Can you work these out from the model? Positions are in its coordinate system, mm. A direction names the side the tool comes from. Round coordinates to 2 decimals unless told otherwise and drop trailing zeros. Write each loop counter-clockwise with the first axis right and the second up, starting at its lowest first coordinate (ties: lowest second). Pieces come first, ordered by that corner, then holes. Notation, with made-up numbers: M 20,22 L 76,22 A3 cw 76,26 Z; hole C 54,53.25 d9. An arc over 180 degrees is marked long. Answer in a Markdown table with one row per item. Add a question column.
(1) Suppose I cut it at A-A, the plane z = 0. Write out the boundary of the cut face in (x, y), then the cut area to 3 significant figures.
(2) Suppose I cut it at D-D, the plane x = -1. Write out the boundary of the cut face in (y, z).
(3) If I drill on probe 1 along Y at (x, z) = (-37.5, 4); probe 2 along X at (y, z) = (-29, 13.5); probe 3 along X at (y, z) = (65, -5), over which ranges is the centre line in solid material (lowest first)?
(4) Suppose I cut it at C-C, the plane y = -27. Write out the boundary of the cut face in (x, z).
(5) I'm going to push flat-ended pins straight in: pin 1 (1.8 mm diameter, centred on x = -2, y = 74, fed in from +Z); pin 2 (3 mm diameter, centred on x = -27.5, z = 5.5, fed in from -Y); pin 3 (6.5 mm diameter, centred on x = -44, y = -30.5, fed in from +Z); pin 4 (12 mm diameter, centred on x = -20.5, z = 24.5, fed in from -Y). Where does each tip first touch, or does it pass through?
(6) For faces 1 (the face through (-40, -13, 15.25)), 2 (the face through (-35, 10.571, 0)), 3 (the face through (-12, -13.5, 0)), which set-ups out of +Z, -Z, +X, -X, +Y, -Y let a thin tool reach every point of the face, with its end or its side?
(7) If we mould it in two halves opening along Z, with no side actions, what happens to faces 4 (the face through (-46, -26, -13.75)), 5 (the face through (-33, -25, 0)), 6 (the face through (0, 74, 10))? For each: released by +Z, released by -Z, zero draft, split by the parting line, or undercut.
(8) Suppose I cut it at B-B, the plane x = -49. Write out the boundary of the cut face in (y, z), then the cut area to 3 significant figures.
from build123d import *

# Parameters (mm, degrees)
SKETCH1_W            = 15
SKETCH1_H            = 18.5
BOSS_EXTRUDE1_DEPTH  = 10
SKETCH3_W            = 60
SKETCH3_H            = 24.642135624
BOSS_EXTRUDE2_DEPTH  = 20
BOSS_EXTRUDE3_DEPTH  = 20
SKETCH5_R            = 5.1
CUT_EXTRUDE1_DEPTH   = 120.21693154
SKETCH6_W            = 15
SKETCH6_H            = 18.5
BOSS_EXTRUDE4_DEPTH  = 50
BOSS_EXTRUDE5_DEPTH  = 25
SKETCH8_W            = 3
SKETCH8_H            = 30.5
BOSS_EXTRUDE6_DEPTH  = 25
SKETCH9_W            = 25
SKETCH9_H            = 1.5
BOSS_EXTRUDE7_DEPTH  = 22
BOSS_EXTRUDE11_START = 2
BOSS_EXTRUDE11_DEPTH = 2


with BuildPart() as part:
    # Sketch1 → Boss-Extrude1 (new, symmetric)
    with BuildSketch(Plane.YZ):
        with BuildLine():
            Line((13.5, 5.25), (13.5, -5.25))
            ThreePointArc((13.5, -5.25), (10.571067812, -12.321067812), (3.5, -15.25))
            Line((3.5, -15.25), (-3.5, -15.25))
            ThreePointArc((-3.5, -15.25), (-10.571067812, -12.321067812), (-13.5, -5.25))
            Line((-13.5, -5.25), (-13.5, 5.25))
            ThreePointArc((-13.5, 5.25), (-10.571067812, 12.321067812), (-3.5, 15.25))
            Line((-3.5, 15.25), (3.5, 15.25))
            ThreePointArc((3.5, 15.25), (10.571067812, 12.321067812), (13.5, 5.25))
        make_face()
        Rectangle(SKETCH1_W, SKETCH1_H, mode=Mode.SUBTRACT)
    extrude(amount=BOSS_EXTRUDE1_DEPTH, both=True)

    # Sketch3 → Boss-Extrude2 (add)
    with BuildSketch(Plane.YZ.offset(10)):
        with Locations((40.571067812, 0)):
            Rectangle(SKETCH3_W, SKETCH3_H)
    extrude(amount=-BOSS_EXTRUDE2_DEPTH)

    # Sketch4 → Boss-Extrude3 (add)
    with BuildSketch(Plane.YZ.offset(10)):
        Polygon((70.571067812, 10), (76.571067812, 10), (76.571067812, 45), (108.571067812, 45), (108.571067812, -45), (76.571067812, -45), (76.571067812, -10), (70.571067812, -10), align=None)
    extrude(amount=-BOSS_EXTRUDE3_DEPTH)

    # Sketch5 → Cut-Extrude1 (cut, through all)
    with BuildSketch(Plane.YZ.offset(10)):
        with Locations(Location((95.921067812, 0, 0), (0, 0, 270))):
            Circle(SKETCH5_R)
    extrude(amount=-CUT_EXTRUDE1_DEPTH, mode=Mode.SUBTRACT)

    # Sketch6 → Boss-Extrude4 (add)
    with BuildSketch(Plane(origin=(-10, 0, 0), x_dir=(0, -1, 0), z_dir=(-1, 0, 0))):
        with BuildLine():
            Line((-10.571067812, 12.321067812), (-10.571067812, -12.321067812))
            ThreePointArc((-10.571067812, -12.321067812), (-7.326834324, -14.488795325), (-3.5, -15.25))
            Line((-3.5, -15.25), (3.5, -15.25))
            ThreePointArc((3.5, -15.25), (10.571067812, -12.321067812), (13.5, -5.25))
            Line((13.5, -5.25), (13.5, 5.25))
            ThreePointArc((13.5, 5.25), (10.571067812, 12.321067812), (3.5, 15.25))
            Line((3.5, 15.25), (-3.5, 15.25))
            ThreePointArc((-3.5, 15.25), (-7.326834324, 14.488795325), (-10.571067812, 12.321067812))
        make_face()
        Rectangle(SKETCH6_W, SKETCH6_H, mode=Mode.SUBTRACT)
    extrude(amount=BOSS_EXTRUDE4_DEPTH)

    # Sketch7 → Boss-Extrude5 (add)
    with BuildSketch(Plane(origin=(-60, 0, 0), x_dir=(0, -1, 0), z_dir=(-1, 0, 0))):
        Polygon((3.5, 15.25), (13.5, 15.25), (13.5, -15.25), (3.5, -15.25), (3.5, -9.25), (7.5, -9.25), (7.5, 9.25), (3.5, 9.25), align=None)
    extrude(amount=-BOSS_EXTRUDE5_DEPTH)

    # Sketch8 → Boss-Extrude6 (add)
    with BuildSketch(Plane.XZ.offset(13.5)):
        with Locations((-58.5, 0)):
            Rectangle(SKETCH8_W, SKETCH8_H)
    extrude(amount=BOSS_EXTRUDE6_DEPTH)

    # Sketch9 → Boss-Extrude7 (add)
    with BuildSketch(Plane.YZ.offset(-57)):
        with Locations((-26, 14.5)):
            Rectangle(SKETCH9_W, SKETCH9_H)
        with Locations((-26, -14.5)):
            Rectangle(SKETCH9_W, SKETCH9_H)
    extrude(amount=BOSS_EXTRUDE7_DEPTH)

    # Sketch10 → Boss-Extrude11 (add)
    with BuildSketch(Plane.YZ.offset(-35).offset(BOSS_EXTRUDE11_START)):
        with BuildLine():
            Line((-3.5, 15.25), (-38.5, 15.25))
            Line((-38.5, 15.25), (-38.5, 13.75))
            Line((-38.5, 13.75), (-13.5, 13.75))
            Line((-13.5, 13.75), (-13.5, 5.25))
            ThreePointArc((-13.5, 5.25), (-10.571067812, 12.321067812), (-3.5, 15.25))
        make_face()
        Polygon((-13.5, 13.75), (-38.5, 13.75), (-38.5, -13.75), (-13.5, -13.75), (-13.5, -5.25), (-13.5, 5.25), align=None)
        with BuildLine():
            Line((-13.5, -13.75), (-38.5, -13.75))
            Line((-38.5, -13.75), (-38.5, -15.25))
            Line((-38.5, -15.25), (-3.5, -15.25))
            ThreePointArc((-3.5, -15.25), (-10.571067812, -12.321067812), (-13.5, -5.25))
            Line((-13.5, -5.25), (-13.5, -13.75))
        make_face()
    extrude(amount=-BOSS_EXTRUDE11_DEPTH)


solid = part.part
Calculated:
| question | item | result |
|---|---|---|
| 1 | outline | M -60,-38.5 L -57,-38.5 L -57,-13.5 L -35,-13.5 L -35,-38.5 L -33,-38.5 L -33,-13.5 L 10,-13.5 L 10,-7.5 L -60,-7.5 Z; M -60,7.5 L 10,7.5 L 10,90.82 L -10,90.82 L -10,10.57 L -60,10.57 Z; M -10,101.02 L 10,101.02 L 10,108.57 L -10,108.57 Z |
| 1 | area | 2,520 mm² |
| 2 | outline | M -13.5,-5.25 A10 ccw -3.5,-15.25 L 3.5,-15.25 A10 ccw 10.57,-12.32 L 70.57,-12.32 L 70.57,-10 L 76.57,-10 L 76.57,-45 L 108.57,-45 L 108.57,45 L 76.57,45 L 76.57,10 L 70.57,10 L 70.57,12.32 L 10.57,12.32 A10 ccw 3.5,15.25 L -3.5,15.25 A10 ccw -13.5,5.25 Z; hole M -7.5,-9.25 L 7.5,-9.25 L 7.5,9.25 L -7.5,9.25 Z; hole C 95.92,0 d10.2 |
| 3 | probe 1 | -13.5 to -7.5, 7.5 to 10.57 |
| 3 | probe 2 | -60 to -57, -35 to -33 |
| 3 | probe 3 | -10 to 10 |
| 4 | outline | M -60,-15.25 L -33,-15.25 L -33,15.25 L -60,15.25 Z; hole M -57,-13.75 L -35,-13.75 L -35,13.75 L -57,13.75 Z |
| 5 | pin 1 | z = 10 |
| 5 | pin 2 | y = -13.5 |
| 5 | pin 3 | z = 15.25 |
| 5 | pin 4 | through |
| 6 | face 1 | +Z, +X, -X, -Y |
| 6 | face 2 | +Z, -Z, -X, +Y |
| 6 | face 3 | +Z, -Z, +X, -Y |
| 7 | face 4 | undercut |
| 7 | face 5 | zero draft |
| 7 | face 6 | released by +Z |
| 8 | outline | M -38.5,-15.25 L 3.5,-15.25 A10 ccw 10.57,-12.32 L 10.57,12.32 A10 ccw 3.5,15.25 L -38.5,15.25 L -38.5,13.75 L -13.5,13.75 L -13.5,-13.75 L -38.5,-13.75 Z; hole M -7.5,-9.25 L 7.5,-9.25 L 7.5,9.25 L -7.5,9.25 Z |
| 8 | area | 519 mm² |
